Verification items for the finished model (mm, model axes). A direction names the side the tool comes from. Give positions to 0.01 mm unless a question says otherwise; leave off trailing zeros. Order: outer loops, then holes, each group sorted by start corner. A loop starts at its lowest first (then second) coordinate and runs counter-clockwise, first axis right, second up.
from build123d import *

# Parameters (mm, degrees)
RIB_DEPTH     = 1
CHAMFER1_SIZE = 1.5


with BuildPart() as part:
    # Sketch1 → Main Body (revolve)
    with BuildSketch(Plane.XY, mode=Mode.PRIVATE) as main_body_sk:
        Polygon((-20, 0), (-20, 8), (-18, 8), (-18, 3.75), (17, 3.75), (17, 3.2), (17.73, 3.2), (17.73, 3.75), (20, 3.75), (20, 0), align=None)
    revolve(main_body_sk.sketch.rotate(Axis((-20, 0, 0), (1, 0, 0)), 90), axis=Axis((-20, 0, 0), (1, 0, 0)))

    # Sketch2 → Rib (add, symmetric)
    with BuildSketch(Plane.XY):
        Polygon((-18, 5.75), (-16, 3.75), (-16, 2.75), (-19, 2.75), (-19, 5.75), align=None)
    extrude(amount=RIB_DEPTH, both=True)

    # Chamfer1
    chamfer1_edges = [part.edges().sort_by_distance(p)[0] for p in [
        (20, 0, -3.75),
    ]]
    chamfer(chamfer1_edges, length=CHAMFER1_SIZE)


solid = part.part
(1) Scan lines: line 1 (X direction, y = 6.75, z = 3.5); line 2 (Y direction, x = 6.5, z = 0); line 3 (Z direction, x = -6.5, y = -3.25). Record each from-to range of solid material in increasing order.
Solved:
line 1: x = -20 to -18
line 2: y = -3.75 to 3.75
line 3: z = -1.87 to 1.87
(2) Set-up check for faces 1 (the flat face through (-17, 4, 1)), 2 (the flat face through (-20, 0, 0)), 3 (the cylindrical face through (18.12, -3.16, 2.02)), 4 (the flat face through (-17, 4, -1)): record each of +Z, -Z, +X, -X, +Y, -Y from which the full face is reachable in a straight line by a thin tool's end or side.
Solved:
face 1: +Z, +X, +Y
face 2: +Z, -Z, -X, +Y, -Y
face 3: +X
face 4: -Z, +X, +Y
(3) Go/stop test with flat-tipped pins: pin 1 (4 mm diameter, centred on x = -15.5, z = -3, fed in from +Y); pin 2 (4 mm diameter, centred on x = -0.5, z = -6.5, fed in from -Y); pin 3 (4 mm diameter, centred on x = -11.5, y = -4, fed in from +Z); pin 4 (4 mm diameter, centred on x = -11.5, y = -5, fed in from +Z). Record where each tip stops, or that it passes through.
Solved:
pin 1: stops at y = 3.61
pin 2: passes through
pin 3: stops at z = 3.17
pin 4: stops at z = 2.25
(4) Section check A-A, the plane y = 0. Enter the section's corners in (x, z).
Solved:
outline: (-20, -8) - (-18, -8) - (-18, -3.75) - (17, -3.75) - (17, -3.2) - (17.73, -3.2) - (17.73, -3.75) - (18.5, -3.75) - (20, -2.25) - (20, 2.25) - (18.5, 3.75) - (17.73, 3.75) - (17.73, 3.2) - (17, 3.2) - (17, 3.75) - (-18, 3.75) - (-18, 8) - (-20, 8) - close
(5) Section check B-B, the plane x = -8. Enter the section's corners in (y, z), then the cut area to 3 significant figures.
Solved:
outline: circle Ø7.5 at (0, 0)
area: 44.2 mm2
(6) Section check C-C, the plane z = 5. Enter the section's corners in (x, y) (3 decimals).
Solved:
outline: (-20, -6.245) - (-18, -6.245) - (-18, 6.245) - (-20, 6.245) - close
(7) Section check D-D, the plane y = 6.5. Enter the section's corners in (x, z), then the cut area to 3 significant figures.
Solved:
outline: (-20, -4.66) - (-18, -4.66) - (-18, 4.66) - (-20, 4.66) - close
area: 18.7 mm2
(8) Release check for a two-part mould opening along X. For faces 5 (the cylindrical face through (-18.99, 7.81, -1.73)), 6 (the flat face through (-17.01, 4.76, 0.01)), 7 (the cylindrical face through (17.37, -0.961, 3.052)) record: pulls with the +X half, pulls with the -X half, needs draft (parallel to the pull), parting line crosses it, or undercut.
Solved:
face 5: needs draft
face 6: pulls with the +X half
face 7: undercut
